Check sheet for the modelled part. Datum: model origin and axes. Units: mm. Face numbers are marked on the shaded views. A direction names the side the tool comes from. Coordinates: 2 decimals unless noted, no trailing zeros. Order: outer loops, then holes, each group sorted by start corner. A loop starts at its lowest first (then second) coordinate and runs counter-clockwise, first axis right, second up.
1. Cross-section at A-A (x = -75.15). Enter the section's corners in (y, z), then the cut area to 3 significant figures.
2. Cross-section at B-B (x = 56). Enter the section's corners in (y, z).
3. Set-up check for the marked faces 4, 5 and 6: record each of +Z, -Z, +X, -X, +Y, -Y from which the full face is reachable in a straight line by a thin tool's end or side.
4. Thickness scan on line 1 (Y direction, x = -77, z = 7); line 2 (Y direction, x = -75.15, z = 1.9); line 3 (X direction, y = 21.5, z = 12). Record the ranges inside material, lowest first.
5. Draft check along Y on the marked faces 1, 2 and 3. Enter one of: released by +Y, released by -Y, zero draft, split by the parting line, or undercut.
6. Gauge pin test, flat ends, axial feed: pin 1 Ø1 at (x, z) = (12, 13) entering from -Y (3 decimals); pin 2 Ø1 at (x, z) = (-55, 14) entering from +Y; pin 3 Ø5 at (y, z) = (29.5, 3.5) entering from -X (3 decimals). Record the tip position at first contact, or that the pin passes through.
7. Cross-section at D-D (y = -1). Enter the section's corners in (x, z).
```python
from build123d import *

# Parameters (mm, degrees)
SKETCH_10_R     = 1.65
EXTRUDE_1_DEPTH = 3
EXTRUDE_START   = 3
EXTRUDE_2_DEPTH = 7
EXTRUDE_3_DEPTH = 13
CHAMFER_1_SIZE  = 7
EXTRUDE_5_DEPTH = 10
FILLET_1_R      = 1


with BuildPart() as part:
    # 草图10 → 凸台-拉伸1 (new body)
    with BuildSketch(Plane.XY):
        Polygon((-85.15, -18.05), (-31.485028843, -18.05), (23.614971157, 37.05), (85.15, 37.05), (85.15, 18.05), (31.485028843, 18.05), (-23.614971157, -37.05), (-85.15, -37.05), align=None)
        with Locations((-75.15, -27.55)):
            Circle(SKETCH_10_R, mode=Mode.SUBTRACT)
        with Locations((75.15, 27.55)):
            Circle(SKETCH_10_R, mode=Mode.SUBTRACT)
    extrude(amount=EXTRUDE_1_DEPTH)

    # 草图11 → 凸台-拉伸2 (add)
    with BuildSketch(Plane.XY.offset(EXTRUDE_START)):
        Polygon((-66.15, -18.05), (-66.15, -37.05), (-23.614971157, -37.05), (31.485028843, 18.05), (66.15, 18.05), (66.15, 37.05), (23.614971157, 37.05), (-31.485028843, -18.05), align=None)
    extrude(amount=EXTRUDE_2_DEPTH)

    # 草图12 → 凸台-拉伸3 (add)
    with BuildSketch(Plane.XY.offset(EXTRUDE_START)):
        Polygon((-85.15, -18.05), (-31.485028843, -18.05), (23.614971157, 37.05), (85.15, 37.05), (85.15, 34.05), (24.857611845, 34.05), (-30.242388155, -21.05), (-85.15, -21.05), align=None)
        Polygon((-85.15, -34.05), (-85.15, -37.05), (-23.614971157, -37.05), (31.485028843, 18.05), (85.15, 18.05), (85.15, 21.05), (30.242388155, 21.05), (-24.857611845, -34.05), align=None)
    extrude(amount=EXTRUDE_3_DEPTH)

    # 倒角1
    chamfer_1_edges = [part.edges().sort_by_distance(p)[0] for p in [
        (66.15, 27.55, 10),
        (-66.15, -27.55, 10),
    ]]
    chamfer(chamfer_1_edges, length=CHAMFER_1_SIZE - 0.0001)  # a hair under: the kernel refuses the full size

    # 草图15 → 凸台-拉伸5 (add)
    with BuildSketch(Plane.XY.offset(3)):
        Polygon((-62.15, -21.05), (-62.15, -25.05), (-28.585533906, -25.05), (26.514466094, 30.05), (62.15, 30.05), (62.15, 34.05), (24.857611845, 34.05), (-30.242388155, -21.05), align=None)
        Polygon((-62.15, -30.05), (-62.15, -34.05), (-24.857611845, -34.05), (30.242388155, 21.05), (62.15, 21.05), (62.15, 25.05), (28.585533906, 25.05), (-26.514466094, -30.05), align=None)
    extrude(amount=EXTRUDE_5_DEPTH)

    # 圆角1
    fillet_1_edges = [part.edges().sort_by_distance(p)[0] for p in [
        (-31.485028843, -18.05, 8),
        (23.614971157, 37.05, 8),
        (31.485028843, 18.05, 8),
        (-23.614971157, -37.05, 8),
        (-28.585533906, -25.05, 11.5),
        (26.514466094, 30.05, 11.5),
        (-26.514466094, -30.05, 11.5),
        (28.585533906, 25.05, 11.5),
        (24.857611845, 34.05, 14.5),
        (-30.242388155, -21.05, 14.5),
        (-24.857611845, -34.05, 14.5),
        (30.242388155, 21.05, 14.5),
    ]]
    fillet(fillet_1_edges, radius=FILLET_1_R)


solid = part.part
```
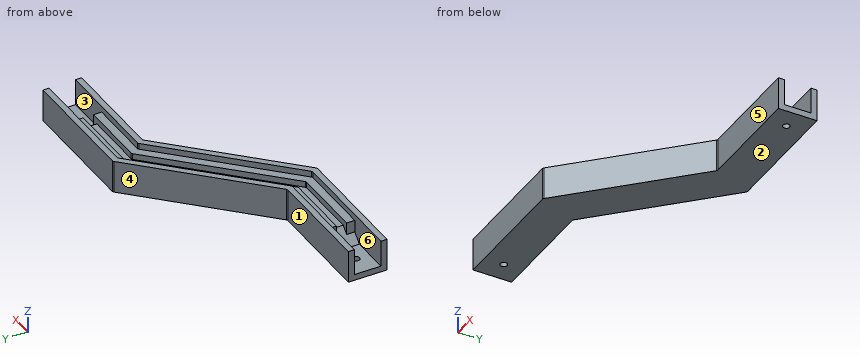
Data:
1. outline: (-37.05, 0) - (-29.2, 0) - (-29.2, 3) - (-34.05, 3) - (-34.05, 16) - (-37.05, 16) - close; (-25.9, 0) - (-18.05, 0) - (-18.05, 16) - (-21.05, 16) - (-21.05, 3) - (-25.9, 3) - close
1. area: 125 mm2
2. outline: (18.05, 0) - (37.05, 0) - (37.05, 16) - (34.05, 16) - (34.05, 13) - (30.05, 13) - (30.05, 10) - (25.05, 10) - (25.05, 13) - (21.05, 13) - (21.05, 16) - (18.05, 16) - close
3. face 4: +Z, -Z, -X, +Y
3. face 5: +Z, -Z, +X, -Y
3. face 6: +Z, -X
4. line 1: y = -37.05 to -34.05, -21.05 to -18.05
4. line 2: y = -37.05 to -29.2, -25.9 to -18.05
4. line 3: x = 8.06 to 17.96, 25.04 to 62.15
5. face 1: released by +Y
5. face 2: zero draft
5. face 3: undercut
6. pin 1: stops at y = -1.935
6. pin 2: stops at y = -18.05
6. pin 3: stops at x = 13.565
7. outline: (-14.44, 0) - (12.44, 0) - (12.44, 16) - (8.19, 16) - (8.19, 13) - (2.54, 13) - (2.54, 10) - (-4.54, 10) - (-4.54, 13) - (-10.19, 13) - (-10.19, 16) - (-14.44, 16) - close
